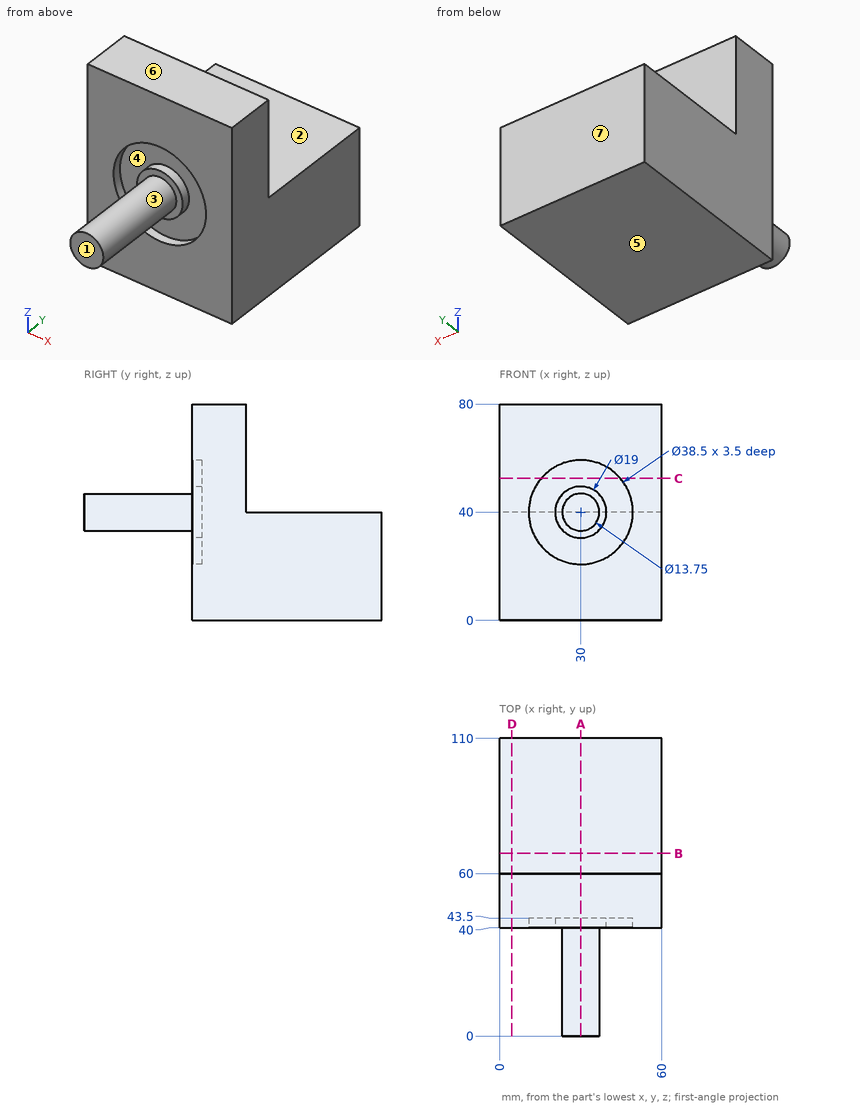
The drawing under review shows one solid part. Ordinate dimensions are in mm from its lowest x, y, z. A direction names the side the tool comes from. Coordinates: 2 decimals unless noted, no trailing zeros. Order: outer loops, then holes, each group sorted by start corner. A loop starts at its lowest first (then second) coordinate and runs counter-clockwise, first axis right, second up. Notation, with made-up numbers: M 54.5,18.25 L 84.5,18.25 A36 ccw 84.5,54.25 Z; hole C -31.5,-30 d10. An arc over 180 degrees is marked long. One line per question, with ' | ' between items.
(1) For probe 1 along Z at (x, y) = (30, 41.95); probe 2 along Y at (x, z) = (50, 47); probe 3 along Z at (x, y) = (36.5, 105), list the stretches that pass through material, from the lowest coordinate up. Write a range as from..to.
Geometry results:
probe 1: z = 0..20.75, 30.5..49.5, 59.25..80 | probe 2: y = 40..60 | probe 3: z = 0..40
(2) The part is to be moulded in two halves that separate along Z. For the marked faces 4, 5, 6 and 7, say which applies: +Z half, -Z half, draft (parallel to the pull), parting line (faces both ways), or undercut.
Geometry results:
face 4: undercut | face 5: -Z half | face 6: +Z half | face 7: draft
(3) Add section D-D, the plane x = 4.5. Write out the cut boundary in (y, z), then the cut area to 3 significant figures.
Geometry results:
outline: M 40,0 L 110,0 L 110,40 L 60,40 L 60,80 L 40,80 Z | area: 3,600 mm²
(4) Add section A-A, the plane x = 30. Write out the cut boundary in (y, z) (3 decimals).
Geometry results:
outline: M 0,33.125 L 40,33.125 L 40,30.5 L 43.5,30.5 L 43.5,20.75 L 40,20.75 L 40,0 L 110,0 L 110,40 L 60,40 L 60,80 L 40,80 L 40,59.25 L 43.5,59.25 L 43.5,49.5 L 40,49.5 L 40,46.875 L 0,46.875 Z
(5) Insertion check: pin 1 (20 mm diameter, centred on x = 29, z = 61, fed in from +Y); pin 2 (3 mm diameter, centred on y = 31.5, z = 47, fed in from +X) (3 decimals); pin 3 (12 mm diameter, centred on y = 73, z = 32.5, fed in from -X); pin 4 (11.5 mm diameter, centred on x = 21, z = 49, fed in from -Y). Each pin has a flat end and moves straight along its axis. Give the tip position at first contact, or say it passes through.
Geometry results:
pin 1: stops at y = 60 | pin 2: stops at x = 34.125 | pin 3: stops at x = 0 | pin 4: stops at y = 40
(6) Add section C-C, the plane z = 52.5. Write out the cut boundary in (x, y), then the cut area to 3 significant figures.
Geometry results:
outline: M 0,40 L 15.36,40 L 15.36,43.5 L 44.64,43.5 L 44.64,40 L 60,40 L 60,60 L 0,60 Z | area: 1,100 mm²
(7) Add section B-B, the plane y = 67.5. Write out the cut boundary in (x, z), then the cut area to 3 significant figures.
Geometry results:
outline: M 0,0 L 60,0 L 60,40 L 0,40 Z | area: 2,400 mm²
(8) Machinability: for the marked faces 1, 2 and 3, which of the approach directions +Z, -Z, +X, -X, +Y, -Y give a long, thin tool a straight path to every point of the face, cutting with its end or side? Answer none if there is none.
Geometry results:
face 1: +Z, -Z, +X, -X, -Y | face 2: +Z, +X, -X, +Y | face 3: -Y
